Could you check a few things on this model? Use its own coordinates, in mm. A direction names the side the tool comes from. Coordinates: 2 decimals unless noted, no trailing zeros. Order: outer loops, then holes, each group sorted by start corner. A loop starts at its lowest first (then second) coordinate and runs counter-clockwise, first axis right, second up. Notation, with made-up numbers: (88.25, 61) - (125.25, 61) arc R34 cw to (125.25, 95) - close; hole circle Ø6 at (61.25, -12). An arc over 180 degrees is marked (long way). Answer as a JSON object with one key per item and string values. Group by question number.
(1) Which directions (+Z, -Z, +X, -X, +Y, -Y) give clear straight access to the entire face, cutting with the end or side of a thin tool? Please do faces 1 (the flat face through (0, 5.5, -7)), 2 (the cylindrical face through (2, 4, 23)).
(2) Please list where these lines run through material, in increasing order: probe 1 along X at (y, z) = (5.5, 22.9); probe 2 along Z at (x, y) = (-1, 4.25); probe 3 along X at (y, z) = (5.5, 22.65).
(3) Will these pins go through, and if not, where does the flat tip stop? P1, Ø3.5, axis at x = 2, y = 5.5, coming from the -Z side; P2, Ø1, axis at x = 8.5, y = 2, coming from the +Z side; P3, Ø2, axis at x = -13, y = 7, coming from the -Z side; P4, Ø3, axis at x = -10, z = -8.5, coming from the -Y side.
(4) We'd pull the mould along X, two halves only. Please class faces 3 (the cylindrical face through (-7.509, 4.451, -23.846)), 4 (the flat face through (0, 5.5, 8)), 5 (the flat face through (0, 0, 0)): pulls with the +X half, pulls with the -X half, needs draft (parallel to the pull), parting line crosses it, or undercut.
(5) Imagine slicing it at A-A, the plane y = 1.75. Write out the boundary of the cut face in (x, z), and give its area (3 significant figures).
from build123d import *

# Parameters (mm, degrees)
CUT_EXTRUDE1_REACH  = 58.471
SKETCH5_R           = 1.5
SKETCH6_R           = 1.5
BOSS_EXTRUDE1_DEPTH = 2.5


with BuildPart() as part:
    # Sketch3 → Revolve3 (revolve)
    with BuildSketch(Plane.XY, mode=Mode.PRIVATE) as revolve3_sk:
        with BuildLine():
            Line((-23, 0), (0, 0))
            Line((0, 0), (0, 3))
            Line((0, 3), (-19.171572875, 3))
            ThreePointArc((-19.171572875, 3), (-19.93693974, 3.152240935), (-20.585786438, 3.585786438))
            Line((-20.585786438, 3.585786438), (-25, 8))
            Line((-25, 8), (-25, 1))
            ThreePointArc((-25, 1), (-24.707106781, 0.292893219), (-24, 0))
            Line((-24, 0), (-23, 0))
        make_face()
    revolve(revolve3_sk.sketch.rotate(Axis((0, 0, 0), (0, 1, 0)), 270), axis=Axis((0, 0, 0), (0, 1, 0)))

    # Cut-Extrude1: up to this cone (the profile starts outside it)
    cut_extrude1_end = Plane(origin=(0, 5.5, 0), z_dir=(0, 1, 0)).offset(-22.499999) * Cone(1e-06, 103.971, 103.970999, align=(Align.CENTER, Align.CENTER, Align.MIN), mode=Mode.PRIVATE)
    # Sketch5 → Cut-Extrude1 (cut, up to the surface)
    with BuildSketch(Plane.XY.offset(25), mode=Mode.PRIVATE) as cut_extrude1_sk1:
        with Locations((-2, 5.5)):
            Circle(SKETCH5_R)
    cut_extrude1_tool1 = extrude(cut_extrude1_sk1.sketch, amount=-CUT_EXTRUDE1_REACH, mode=Mode.PRIVATE) - cut_extrude1_end
    add(cut_extrude1_tool1.solids().sort_by_distance((-2, 5.5, 25))[0], mode=Mode.SUBTRACT)
    # Sketch5 → Cut-Extrude1 (cut, up to the surface)
    with BuildSketch(Plane.XY.offset(25), mode=Mode.PRIVATE) as cut_extrude1_sk2:
        with Locations((2, 5.5)):
            Circle(SKETCH5_R)
    cut_extrude1_tool2 = extrude(cut_extrude1_sk2.sketch, amount=-CUT_EXTRUDE1_REACH, mode=Mode.PRIVATE) - cut_extrude1_end
    add(cut_extrude1_tool2.solids().sort_by_distance((2, 5.5, 25))[0], mode=Mode.SUBTRACT)

    # Sketch6 → Boss-Extrude1 (add)
    with BuildSketch(Plane(origin=(0, 3, 0), x_dir=(1, 0, 0), z_dir=(0, 1, 0))):
        with Locations(Location((0, 7.5, 0), (0, 0, 90))):
            Circle(SKETCH6_R)
        with Locations(Location((0, -7.5, 0), (0, 0, 90))):
            Circle(SKETCH6_R)
    extrude(amount=BOSS_EXTRUDE1_DEPTH)


solid = part.part
Result set:
{
 "1": {"face 1": "+Y", "face 2": "+Z"},
 "2": {"probe 1": "x = -10.03 to -3.5, -0.5 to 0.5, 3.5 to 10.03", "probe 2": "z = -24.98 to -21.23, -8.62 to -6.38, 6.38 to 8.62, 21.23 to 24.98", "probe 3": "x = -10.58 to -3.5, -0.5 to 0.5, 3.5 to 10.58"},
 "3": {"P1": "stops at z = -25", "P2": "stops at z = 23.69", "P3": "stops at z = -21.93", "P4": "stops at y = 0"},
 "4": {"face 3": "parting line crosses it", "face 4": "undercut", "face 5": "needs draft"},
 "5": {"outline": "circle Ø50 at (0, 0)", "area": "1,960 mm^2"}
}
